Build history of the part. All positions in model axes, mm. A direction names the side the tool comes from. Coordinates: 2 decimals unless noted, no trailing zeros. Write each loop counter-clockwise with the first axis right and the second up, starting at its lowest first coordinate (ties: lowest second). Pieces come first, ordered by that corner, then holes. Notation, with made-up numbers: (13.5, 51.5) -> (55.5, 51.5) arc R21 ccw to (55.5, 63.5) -> close; hole circle Ø5 at (45.25, -28.75). An arc over 180 degrees is marked (long way). Write each question's results on one line, items separated by ' | '. Start each with the question number.
Q1. Saw through at D-D on x = 35. Give the cut face in (y, z), and give its area (3 significant figures).
Q2. Drill centre lines: line 1 (X direction, y = 7, z = 1.6); line 2 (X direction, y = 7.75, z = 2.5); line 3 (Y direction, x = 7, z = 3.45). Where is each one in solid material? Low to high.
Q3. Tool access for faces 1 (the face through (42, 7, 3)), 2 (the face through (5, 9, 6)), 3 (the face through (27.5, 7, 19)): list every direction of +Z, -Z, +X, -X, +Y, -Y with a clear straight run to the whole face (end or side of a thin tool).
Q4. Drop flat-ended pins along their axis: pin 1 Ø1 at (x, z) = (27, 26.5) entering from -Y; pin 2 Ø5 at (x, y) = (32.5, 4.5) entering from +Z; pin 3 Ø7 at (y, z) = (8, 21.5) entering from +X; pin 4 Ø1 at (x, z) = (37, 7.5) entering from +Y. Give the stop position or say it passes through.
Q5. Saw through at A-A on y = 7. Give the cut face in (x, z).
Q6. Saw through at B-B on z = 20. Give the cut face in (x, y), and give its area (3 significant figures).
Q7. Two-plate mould, pull along Y, no slides. Class faces 4 (the face through (8.21, 8.897, 2.958)), 5 (the face through (13.5, 7, 19)), 6 (the face through (21, 14, 13)), 7 (the face through (20.402, 6.512, 25.804)): released by +Y, released by -Y, zero draft, split by the parting line, or undercut.
Q8. Saw through at C-C on x = 22.5. Give the cut face in (y, z).
from build123d import *

# Parameters (mm, degrees)
CYLINDER003_R       = 2.25
CYLINDER003_DEPTH   = 10
CYLINDER002_R       = 2.25
CYLINDER002_DEPTH   = 10
CYLINDER001_R       = 2.25
CYLINDER001_DEPTH   = 30
CYLINDER_R          = 4.5
CYLINDER_DEPTH      = 30
CYLINDER_ROLL_ANGLE = 90
BOX001_W            = 14
BOX001_H            = 14
BOX001_DEPTH        = 27
BOX_W               = 42
BOX_H               = 14
BOX_DEPTH           = 6


with BuildPart() as cilindro003:
    # Cylinder003 → Cylinder003 (new body)
    with BuildSketch(Plane(origin=(35, 7, 0), x_dir=(1, 0, 0), z_dir=(0, 0, 1))):
        Circle(CYLINDER003_R)
    extrude(amount=CYLINDER003_DEPTH)


with BuildPart() as cilindro002:
    # Cylinder002 → Cylinder002 (new body)
    with BuildSketch(Plane(origin=(7, 7, 0), x_dir=(1, 0, 0), z_dir=(0, 0, 1))):
        Circle(CYLINDER002_R)
    extrude(amount=CYLINDER002_DEPTH)


with BuildPart() as cilindro001:
    # Cylinder001 → Cylinder001 (new body)
    with BuildSketch(Plane(origin=(10, 7, 28), x_dir=(0, 1, 0), z_dir=(1, 0, 0))):
        Circle(CYLINDER001_R)
    extrude(amount=CYLINDER001_DEPTH)


with BuildPart() as cilindro:
    # Cylinder → Cylinder (new body)
    with BuildSketch(Plane.XY):
        Circle(CYLINDER_R)
    extrude(amount=CYLINDER_DEPTH)


with BuildPart() as cilindro_1:
    # Cylinder roll: moved
    add(cilindro.part.rotate(Axis((0, 0, 0), (1, 0, 0)), CYLINDER_ROLL_ANGLE))


with BuildPart() as cilindro_2:
    # Cylinder placement: moved
    add(cilindro_1.part.moved(Location((21.158, 20, 20))))


with BuildPart() as cubo001:
    # Box001 → Box001 (new body)
    with BuildSketch(Plane(origin=(13.5, 0, 6), x_dir=(1, 0, 0), z_dir=(0, 0, 1))):
        with Locations((7, 7)):
            Rectangle(BOX001_W, BOX001_H)
    extrude(amount=BOX001_DEPTH)


with BuildPart() as cut003:
    # Box → Box (new body)
    with BuildSketch(Plane.XY):
        with Locations((21, 7)):
            Rectangle(BOX_W, BOX_H)
    extrude(amount=BOX_DEPTH)

    # Fusion: union Cubo001
    add(cubo001.part)

    # Cut: cut Cilindro
    add(cilindro_2.part, mode=Mode.SUBTRACT)

    # Cut001: cut Cilindro001
    add(cilindro001.part, mode=Mode.SUBTRACT)

    # Cut002: cut Cilindro002
    add(cilindro002.part, mode=Mode.SUBTRACT)

    # Cut003: cut Cilindro003
    add(cilindro003.part, mode=Mode.SUBTRACT)


solid = cut003.part
Returned:
1) outline: (0, 0) -> (4.75, 0) -> (4.75, 6) -> (0, 6) -> close; (9.25, 0) -> (14, 0) -> (14, 6) -> (9.25, 6) -> close | area: 57.0 mm2
2) line 1: x = 0 to 4.75, 9.25 to 32.75, 37.25 to 42 | line 2: x = 0 to 4.88, 9.12 to 32.88, 37.12 to 42 | line 3: y = 0 to 4.75, 9.25 to 14
3) face 1: +Z, -Z, +X, +Y, -Y | face 2: +Z, -X, +Y, -Y | face 3: +Z, +X, +Y, -Y
4) pin 1: stops at y = 0 | pin 2: stops at z = 6 | pin 3: stops at x = 27.5 | pin 4: passes through
5) outline: (0, 0) -> (4.75, 0) -> (4.75, 6) -> (0, 6) -> close; (9.25, 0) -> (32.75, 0) -> (32.75, 6) -> (27.5, 6) -> (27.5, 25.75) -> (13.5, 25.75) -> (13.5, 6) -> (9.25, 6) -> close; (13.5, 30.25) -> (27.5, 30.25) -> (27.5, 33) -> (13.5, 33) -> close; (37.25, 0) -> (42, 0) -> (42, 6) -> (37.25, 6) -> close; hole circle Ø9 at (21.16, 20)
6) outline: (13.5, 0) -> (16.66, 0) -> (16.66, 14) -> (13.5, 14) -> close; (25.66, 0) -> (27.5, 0) -> (27.5, 14) -> (25.66, 14) -> close | area: 70.0 mm2
7) face 4: undercut | face 5: zero draft | face 6: released by +Y | face 7: undercut
8) outline: (0, 0) -> (14, 0) -> (14, 15.7) -> (0, 15.7) -> close; (0, 24.3) -> (14, 24.3) -> (14, 33) -> (0, 33) -> close; hole circle Ø4.5 at (7, 28)
